Read the model definition and answer for the solid it produces. Units are mm, in the model's axes. A direction names the side the tool comes from. Round coordinates to 2 decimals unless told otherwise and drop trailing zeros. Write each loop counter-clockwise with the first axis right and the second up, starting at its lowest first coordinate (ties: lowest second). Pieces come first, ordered by that corner, then holes. Notation, with made-up numbers: (51.25, 67) -> (88.25, 67) arc R35 cw to (88.25, 99) -> close; hole circle Ø7 at (35, 49.5). An arc over 180 degrees is marked (long way). Return JSON: item names as keys, results as strings.
Autodesk Inventor part; units mm, degrees
ref_plane "YZ Plane" through (0, 0, 0) normal (1, 0, 0) x (0, 1, 0)
ref_plane "XZ Plane" through (0, 0, 0) normal (0, 1, 0) x (-1, 0, 0)
ref_plane "XY Plane" through (0, 0, 0) normal (0, 0, 1) x (1, 0, 0)
sketch "Sketch1" plane through (0, 0, 0) normal (0, 1, 0) x (-1, 0, 0)
  line L0 (-276.225, 292.1) -> (-276.225, -292.1)
  line L1 (-276.225, -292.1) -> (276.225, -292.1)
  line L2 (276.225, -292.1) -> (276.225, 292.1)
  line L3 (276.225, 292.1) -> (-276.225, 292.1)
  line L4 (-276.225, 292.1) -> (276.225, -292.1) construction
  line L5 (-276.225, -292.1) -> (276.225, 292.1) construction
  point P0 (0, 0)
  dimension "baseLength" = 584.2
  dimension "baseWidth" = 552.45
extrude "Extrusion1" add sketch "Sketch1" along normal blind 17.78
sketch "Sketch2" plane through (0, 0, 0) normal (0, -1, 0) x (1, 0, 0)
  line L0 (276.225, 292.1) -> (276.225, -292.1)
  line L1 (276.225, 209.55) -> (123.825, 209.55)
  line L2 (123.825, 209.55) -> (123.825, 63.5)
  line L3 (123.825, 63.5) -> (276.225, 63.5)
  line L4 (276.225, 63.5) -> (276.225, 209.55)
  line L5 (-276.225, 292.1) -> (276.225, 292.1)
  point P0 (0, 0)
  dimension "backToEndOfGearBox" = 82.55
  dimension "backToFrontOfGearBox" = 228.6
  dimension "wdithForGearBox" = 152.4
extrude "Extrusion2" cut sketch "Sketch2" against normal through all
mirror "Mirror1" about plane through (0, 0, 0) normal (1, 0, 0) of "Extrusion2"
equation "\"spaceingAlongSides\" = 3.175"
equation "\"distanceFromBackForEndBolt\" = 38.1"
equation "\"spacingForBolt\" = 25.4"
equation "\"widthOfSpacingForBolt\" = 12.7"
equation "\"lengthOfSpacingForBolt\" = 25.4"
properties part number "RhinoBottomFloorPlate03" material "Wood (Birch)"
Item 1: Straight lines are drawn through the part: L1, parallel to Z at x = 155, y = 8.75; L2, parallel to X at y = 16.5, z = 182.5 (3 decimals). For each, find the intervals that lie inside material, in ascending order. Write a range as [from, to].
Worked answers:
{"L1": "z = [-292.1, 63.5], [209.55, 292.1]", "L2": "x = [-123.825, 123.825]"}
Item 2: A tool of negligible diameter and unlimited length cuts with its end or side. For faces 4 (the flat face through (-199, 9, 209.55)), 5 (the flat face through (123.825, 9, 138)), 6 (the flat face through (-276.225, 9, -117)), from which of +Z, -Z, +X, -X, +Y, -Y can it reach the whole face along a straight path? Write none if from no direction.
Worked answers:
{"face 4": "-X, +Y, -Y", "face 5": "+X, +Y, -Y", "face 6": "+Z, -Z, -X, +Y, -Y"}
Item 3: A flat-ended cylindrical pin translates along its axis: pin 1 (5.5 mm diameter, centred on y = 11.5, z = 111, fed in from +X) (3 decimals). Find the tip coordinate at first contact, or state that the pin passes through.
Worked answers:
{"pin 1": "stops at x = 123.825"}
Item 4: Section A-A (x = -216.5) is taken. Give the vertices of the cut face in (y, z).
Worked answers:
{"outline": "(0, -292.1) -> (17.78, -292.1) -> (17.78, 63.5) -> (0, 63.5) -> close; (0, 209.55) -> (17.78, 209.55) -> (17.78, 292.1) -> (0, 292.1) -> close"}
Item 5: Section B-B (y = 9.5) is taken. Give the vertices of the cut face in (x, z) (3 decimals), then the cut area to 3 significant figures.
Worked answers:
{"outline": "(-276.225, -292.1) -> (276.225, -292.1) -> (276.225, 63.5) -> (123.825, 63.5) -> (123.825, 209.55) -> (276.225, 209.55) -> (276.225, 292.1) -> (-276.225, 292.1) -> (-276.225, 209.55) -> (-123.825, 209.55) -> (-123.825, 63.5) -> (-276.225, 63.5) -> close", "area": "278,000 mm2"}
Item 6: For a pull along Z with two mould halves and no side action, classify faces 1 (the flat face through (4, 9, -292.1)), 2 (the flat face through (276.225, 9, -112)), 3 (the flat face through (-201, 9, 63.5)) as released by +Z, released by -Z, zero draft, split by the parting line, or undercut.
Worked answers:
{"face 1": "released by -Z", "face 2": "zero draft", "face 3": "undercut"}
Item 7: Section C-C (z = 78.5) is taken. Give the vertices of the cut face in (x, y) (3 decimals).
Worked answers:
{"outline": "(-123.825, 0) -> (123.825, 0) -> (123.825, 17.78) -> (-123.825, 17.78) -> close"}
